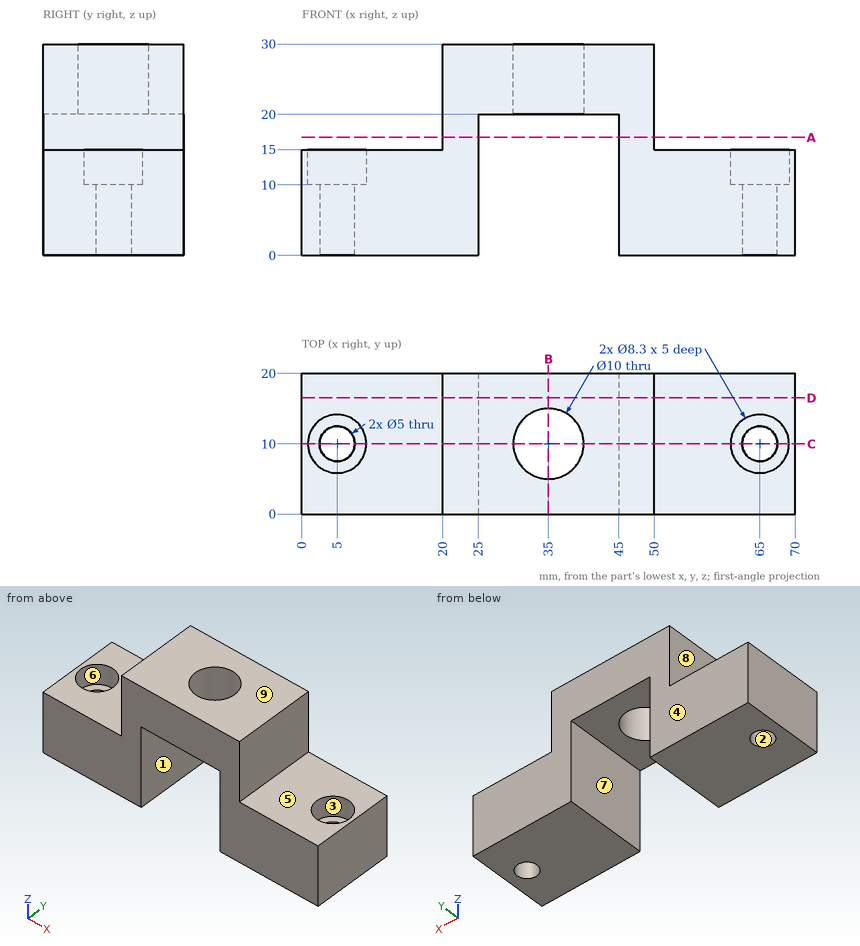
Could you check a few things on this drawing? It's one solid part, dimensions in mm from its lowest x, y, z. A direction names the side the tool comes from. Give positions to 0.01 mm unless a question says otherwise; leave off trailing zeros. Order: outer loops, then holes, each group sorted by start corner. A loop starts at its lowest first (then second) coordinate and runs counter-clockwise, first axis right, second up. Notation, with made-up numbers: (-10, -15) - (44, -15) arc R17 ccw to (44, 12) - close; hole circle Ø11 at (-2.5, 2). An arc over 180 degrees is marked (long way). Return JSON: item names as keys, results as strings. Group by question number.
Q1. Will these pins go through, and if not, where does the flat tip stop? pin 1 Ø3 at (y, z) = (4.5, 20.5) entering from +X; pin 2 Ø1 at (y, z) = (9, 15) entering from -X; pin 3 Ø9 at (x, y) = (65.5, 10) entering from +Z; pin 4 Ø12 at (y, z) = (6, 22) entering from -X.
Q2. Thinking about a two-plate mould opening in Y: for the marked faces 1, 2, 3 and 4, which applies, pulls with the +Y half, pulls with the -Y half, needs draft (parallel to the pull), parting line crosses it, or undercut?
Q3. Suppose I cut it at B-B, the plane x = 35. Please give me the cut outline in (y, z), and give its area (3 significant figures).
Q4. Suppose I cut it at D-D, the plane y = 16.5. Please give me the cut outline in (x, z).
Q5. Suppose I cut it at A-A, the plane z = 16.75. Please give me the cut outline in (x, y).
Q6. Suppose I cut it at C-C, the plane y = 10. State how many separate pieces and enclosed holes the cut face has, and give its area (3 significant figures).
Q7. Which directions (+Z, -Z, +X, -X, +Y, -Y) give clear straight access to the entire face, cutting with the end or side of a thin tool? Please do the marked faces 5, 6, 7, 8 and 9.
Q8. Please list where these lines run through material, in increasing order: line 1 along X through (y, z) = (10, 3.5); line 2 along Y through (x, z) = (35, 26.25); line 3 along X through (y, z) = (3.25, 3.5). Write a range as [from, to].
Resolved:
{
 "1": {"pin 1": "stops at x = 50", "pin 2": "stops at x = 0", "pin 3": "stops at z = 15", "pin 4": "stops at x = 20"},
 "2": {"face 1": "needs draft", "face 2": "undercut", "face 3": "undercut", "face 4": "pulls with the +Y half"},
 "3": {"outline": "(0, 20) - (5, 20) - (5, 30) - (0, 30) - close; (15, 20) - (20, 20) - (20, 30) - (15, 30) - close", "area": "100 mm2"},
 "4": {"outline": "(0, 0) - (25, 0) - (25, 20) - (45, 20) - (45, 0) - (70, 0) - (70, 15) - (50, 15) - (50, 30) - (20, 30) - (20, 15) - (0, 15) - close"},
 "5": {"outline": "(20, 0) - (25, 0) - (25, 20) - (20, 20) - close; (45, 0) - (50, 0) - (50, 20) - (45, 20) - close"},
 "6": {"separate pieces": "4", "enclosed holes": "0", "area": "817 mm2"},
 "7": {"face 5": "+Z, +X, +Y, -Y", "face 6": "+Z", "face 7": "-Z, +Y, -Y", "face 8": "+Z, -X, +Y, -Y", "face 9": "+Z, +X, -X, +Y, -Y"},
 "8": {"line 1": "x = [0, 2.5], [7.5, 25], [45, 62.5], [67.5, 70]", "line 2": "y = [0, 5], [15, 20]", "line 3": "x = [0, 25], [45, 70]"}
}
